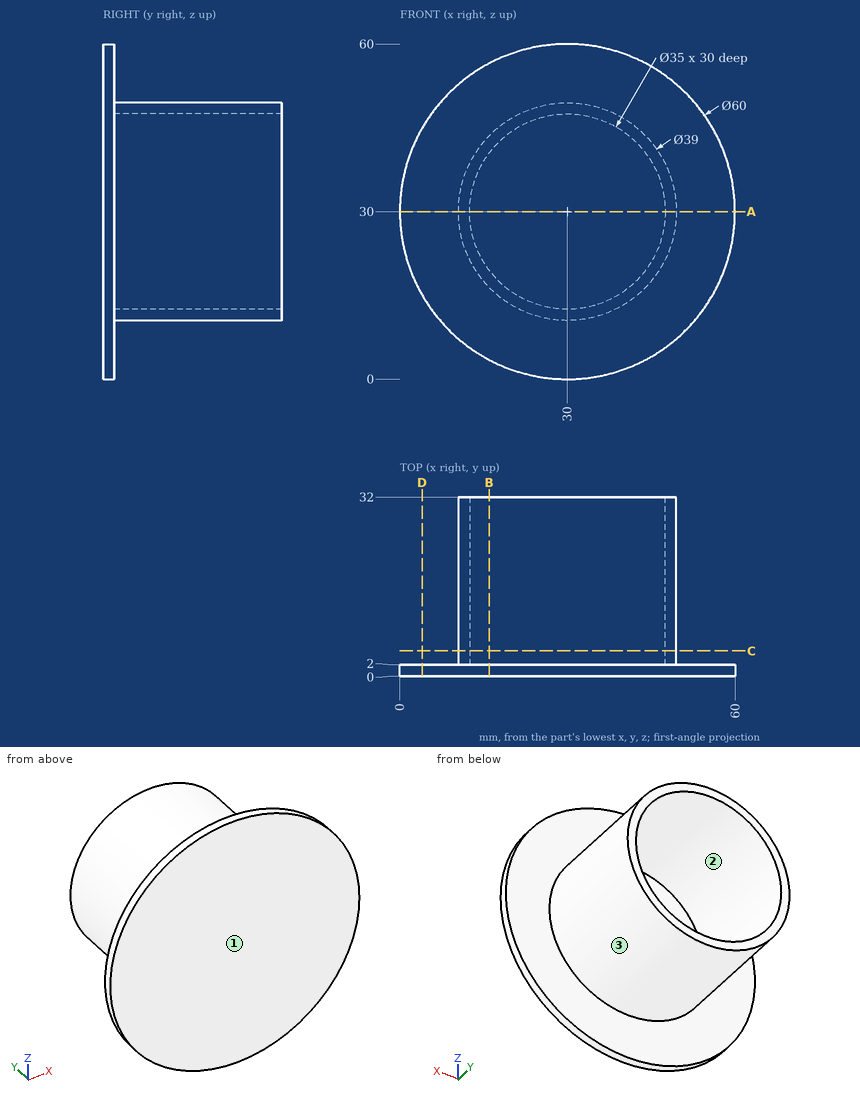
Geometry: see drawing. Coordinates: mm, zero at the bounding-box minimum. Give positions to 0.01 mm unless a question says otherwise; leave off trailing zeros. Loops run counter-clockwise (first coordinate to the right, second up) from the corner with the lowest first, then second, coordinate; pieces in that order, holes last. Notation, with made-up numbers: (-24.5, 82.5) -> (29.5, 82.5) arc R17 cw to (29.5, 105.5) -> close; hole circle Ø8 at (63.5, -35.5). An arc over 180 degrees is marked (long way). Put each result on its own line as item: value.
1. Pull-direction query (Z, two-part tool) for the marked faces 1, 2 and 3; classes: released by +Z, released by -Z, zero draft, split by the parting line, or undercut.
Taken from the geometry:
face 1: zero draft
face 2: undercut
face 3: split by the parting line
2. Cut plane C-C (y = 4.5). Return the cut outline in (x, z).
Taken from the geometry:
outline: circle Ø39 at (30, 30); hole circle Ø35 at (30, 30)
3. Pin query (flat end, axial travel): P1, Ø4, axis at y = 26.5, z = 19, coming from the -X side; P2, Ø4, axis at x = 42, z = 51.5, coming from the -Y side; P3, Ø8, axis at y = 4.5, z = 24, coming from the -X side; P4, Ø12, axis at y = 11, z = 17.5, coming from the +X side. Return the tip coordinate at first contact, or that it passes through.
Taken from the geometry:
P1: stops at x = 12.7
P2: stops at y = 0
P3: stops at x = 0.14
P4: stops at x = 48.38
4. Cut plane B-B (x = 16). Return the cut outline in (y, z).
Taken from the geometry:
outline: (0, 3.47) -> (2, 3.47) -> (2, 16.43) -> (32, 16.43) -> (32, 19.5) -> (2, 19.5) -> (2, 40.5) -> (32, 40.5) -> (32, 43.57) -> (2, 43.57) -> (2, 56.53) -> (0, 56.53) -> close
5. Ray query, line 1 along X through (y, z) = (13, 30); line 2 along Y through (x, z) = (47, 17.5). Return the intervals inside material, ascending. Write a range as [from, to].
Taken from the geometry:
line 1: x = [10.5, 12.5], [47.5, 49.5]
line 2: y = [0, 2]
6. Cut plane A-A (z = 30). Return the cut outline in (x, y), plus the area to 3 significant figures.
Taken from the geometry:
outline: (0, 0) -> (60, 0) -> (60, 2) -> (49.5, 2) -> (49.5, 32) -> (47.5, 32) -> (47.5, 2) -> (12.5, 2) -> (12.5, 32) -> (10.5, 32) -> (10.5, 2) -> (0, 2) -> close
area: 240 mm2
7. Cut plane D-D (x = 4). Return the cut outline in (y, z).
Taken from the geometry:
outline: (0, 15.03) -> (2, 15.03) -> (2, 44.97) -> (0, 44.97) -> close
